For this review, use the dimensioned drawing (mm, ordinates from the lowest corner) and the shaded views. Coordinates: 2 decimals unless noted, no trailing zeros. Loops run counter-clockwise (first coordinate to the right, second up) from the corner with the lowest first, then second, coordinate; pieces in that order, holes last. Notation, with made-up numbers: (76.5, -35) - (126.5, -35) arc R21 cw to (126.5, -20) - close; hole circle Ø9 at (-16, 19). An arc over 180 degrees is marked (long way). Answer in a Markdown table with one row per item. Add a question column.
(1) We need section B-B, the plane x = 20. Write out the cut boundary in (y, z).
(2) To check wall thickness, follow L1, parallel to X at y = 319.5, z = 13.25; L2, parallel to Y at x = 20, z = 17.5; L3, parallel to Y at x = 10, z = 4.25. State the ranges of each line that lie inside material, in increasing order. Write a range as [from, to].
(3) We need section C-C, the plane y = 219.5. Write out the cut boundary in (x, z), plus the area to 3 significant figures.
(4) We need section A-A, the plane y = 320. Write out the cut boundary in (x, z), plus the area to 3 significant figures.
(5) Clearance check with flat-ended pins moving along their axes: pin 1 (3 mm diameter, centred on y = 223.5, z = 9.5, fed in from -X); pin 2 (2 mm diameter, centred on y = 295.5, z = 7.5, fed in from -X); pin 3 (5 mm diameter, centred on y = 209.5, z = 15, fed in from +X). State where each tip first meets the part, or that it passes through.
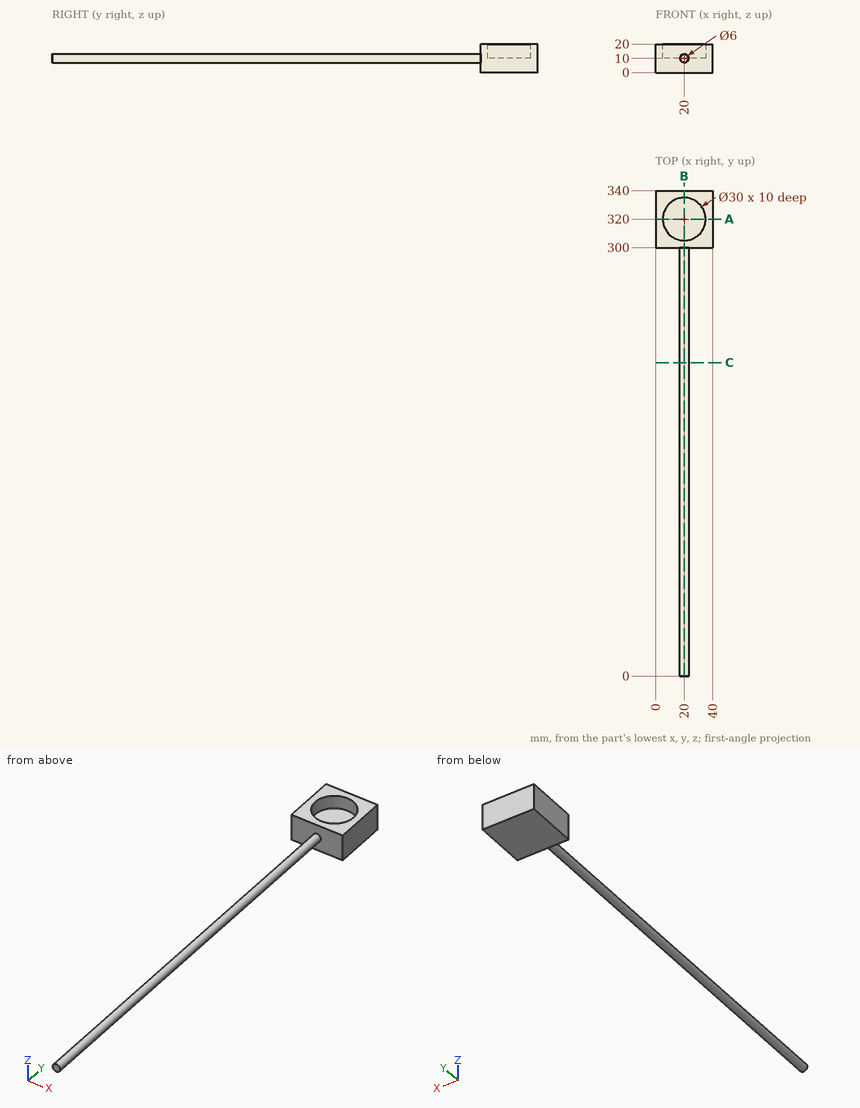
Responses:
| question | item | result |
|---|---|---|
| 1 | outline | (0, 7) - (300, 7) - (300, 0) - (340, 0) - (340, 20) - (335, 20) - (335, 10) - (305, 10) - (305, 20) - (300, 20) - (300, 13) - (0, 13) - close |
| 2 | L1 | x = [0, 5.01], [34.99, 40] |
| 2 | L2 | y = [300, 305], [335, 340] |
| 2 | L3 | y = [300, 340] |
| 3 | outline | circle Ø6 at (20, 10) |
| 3 | area | 28.3 mm2 |
| 4 | outline | (0, 0) - (40, 0) - (40, 20) - (35, 20) - (35, 10) - (5, 10) - (5, 20) - (0, 20) - close |
| 4 | area | 500 mm2 |
| 5 | pin 1 | stops at x = 17 |
| 5 | pin 2 | stops at x = 17.4 |
| 5 | pin 3 | stops at x = 21.66 |
